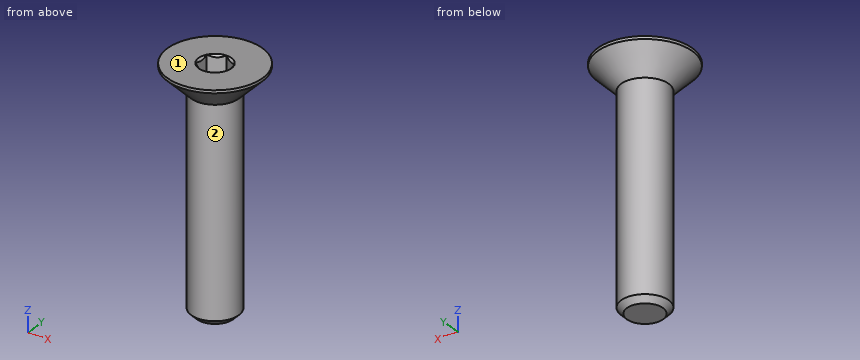
```python
from build123d import *

# Parameters (mm, degrees)
SKETCH1_W          = 25
SKETCH1_H          = 2.5
CHAMFER1_SIZE      = 0.6
CUT_EXTRUDE2_DEPTH = 1.96


with BuildPart() as part:
    # Sketch1 → Revolve1 (revolve)
    with BuildSketch(Plane(origin=(0, 0, 0), x_dir=(0, 0, -1), z_dir=(1, 0, 0))):
        with Locations((12.5, 1.25)):
            Rectangle(SKETCH1_W, SKETCH1_H)
    revolve(axis=Axis((0, 0, -25), (0, 0, 1)))

    # Chamfer1
    chamfer1_edges = [part.edges().sort_by_distance(p)[0] for p in [
        (0, -2.5, -25),
    ]]
    chamfer(chamfer1_edges, length=CHAMFER1_SIZE)

    # Sketch7 → Revolve2 (revolve)
    with BuildSketch(Plane(origin=(0, 0, 0), x_dir=(0, 0, -1), z_dir=(1, 0, 0)), mode=Mode.PRIVATE) as revolve2_sk:
        Polygon((0, 5), (0.3, 5), (2.8, 2.5), (2.8, 0), (0, 0), align=None)
    revolve(revolve2_sk.sketch.rotate(Axis((0, 0, 0), (0, 0, -1)), 180), axis=Axis((0, 0, 0), (0, 0, -1)))

    # Boss-Extrude1 cone 1 section (through the dimple's axis) → Boss-Extrude1 (revolve)
    with BuildSketch(Plane(origin=(0, 0, -2.8), x_dir=(0, -1, 0), z_dir=(1, 0, 0))):
        Polygon((0, 0), (2.5, 0), (0, 2.5), align=None)
    revolve(axis=Axis((0, 0, -2.8), (0, 0, -1)))

    # Sketch5 → Cut-Extrude2 (cut)
    with BuildSketch(Plane.XY):
        Polygon((1.5, -0.866025404), (1.5, 0.866025404), (0, 1.732050808), (-1.5, 0.866025404), (-1.5, -0.866025404), (0, -1.732050808), align=None)
    extrude(amount=-CUT_EXTRUDE2_DEPTH, mode=Mode.SUBTRACT)

    # Cut-Extrude3 cone 1 section (through the dimple's axis) → Cut-Extrude3 (revolve, cut)
    with BuildSketch(Plane(origin=(0, 0, 0), x_dir=(0, -1, 0), z_dir=(1, 0, 0))):
        Polygon((0, 0), (1.732050808, 0), (0, 1.732050808), align=None)
    revolve(axis=Axis((0, 0, 0), (0, 0, -1)), mode=Mode.SUBTRACT)


solid = part.part
```
CAD build for the part. Positions are in the model's coordinates, mm. Face numbers are marked on the shaded views. A direction names the side the tool comes from. Round coordinates to 2 decimals unless told otherwise and drop trailing zeros. Order: outer loops, then holes, each group sorted by start corner. A loop starts at its lowest first (then second) coordinate and runs counter-clockwise, first axis right, second up.
Q1. Slice it at A-A (y = 0). Write the cut outline in (x, z).
Q2. Wall check: L1, parallel to Z at x = -0.25, y = 1.5; L2, parallel to X at y = 2, z = -13.25; L3, parallel to X at y = 0.5, z = -7.25. Give the ranges that are in metal, low to high.
Q3. Which spindle directions (+Z, -Z, +X, -X, +Y, -Y) get a long thin tool onto all of the face, cutting with end or side? Do the marked faces 1 and 2. Say none if no direction does.
Q4. Drop flat-ended pins along their axis: pin 1 (0.5 mm diameter, centred on y = 0, z = -1.5, fed in from +X); pin 2 (3 mm diameter, centred on y = 3.5, z = -17, fed in from -X); pin 3 (3 mm diameter, centred on x = 1, z = -6.5, fed in from +Y); pin 4 (2.5 mm diameter, centred on x = 0.5, y = -0.5, fed in from +Z). Give the stop position or say it passes through.
Q5. Slice it at B-B (z = -20.75). Write the cut outline in (x, y), and give its area (3 significant figures).
Results below:
1. outline: (-5, -0.3) - (-2.5, -2.8) - (-2.5, -24.4) - (-1.9, -25) - (1.9, -25) - (2.5, -24.4) - (2.5, -2.8) - (5, -0.3) - (5, 0) - (1.73, 0) - (1.5, -0.23) - (1.5, -1.96) - (-1.5, -1.96) - (-1.5, -0.23) - (-1.73, 0) - (-5, 0) - close
2. L1: z = -25 to -1.96
2. L2: x = -1.5 to 1.5
2. L3: x = -2.45 to 2.45
3. face 1: +Z, +X, -X, +Y, -Y
3. face 2: -Z
4. pin 1: stops at x = 4.05
4. pin 2: stops at x = -1.5
4. pin 3: stops at y = 2.5
4. pin 4: stops at z = 0
5. outline: circle Ø5 at (0, 0)
5. area: 19.6 mm2
